For this review, take the finished solid that the model builds, in its own axes (mm). Face numbers are marked on the shaded views. A direction names the side the tool comes from. Give positions to 0.01 mm unless a question says otherwise; leave off trailing zeros. Write each loop counter-clockwise with the first axis right and the second up, starting at its lowest first coordinate (ties: lowest second). Pieces come first, ordered by that corner, then holes.
Q1. We need section D-D (z = -11). Write out the cut boundary in (x, y).
Q2. Machinability: for the marked faces 1, 2 and 3, which of the approach directions +Z, -Z, +X, -X, +Y, -Y give a long, thin tool a straight path to every point of the face, cutting with its end or side? Answer none if there is none.
Q3. We need section B-B (y = 0.95). Write out the cut boundary in (x, z).
Q4. For line 1 (X direction, y = 3.8, z = 0); line 2 (Z direction, x = 31.5, y = 2.6); line 3 (X direction, y = 4.75, z = -11.5), list the stretches that pass through material, from the lowest coordinate up.
Q5. We need section A-A (z = 0). Write out the cut boundary in (x, y).
Q6. Mouldability with a two-part tool opening along Z and no side actions: class the marked faces 4, 5, 6 and 7 as released by +Z, released by -Z, zero draft, split by the parting line, or undercut.
Q7. We need section C-C (x = -24). Write out the cut boundary in (y, z), then the cut area to 3 significant figures.
Q8. Insertion check: P1, Ø2.5, axis at y = 3.5, z = 13, coming from the +X side; P2, Ø1.6, axis at x = 33, y = 2, coming from the +Z side; P3, Ø2, axis at x = 32, y = 3.5, coming from the -Z side. Each pin has a flat end and moves straight along its axis. Give the tip position at first contact, or say it passes through.
```python
from build123d import *

# Parameters (mm, degrees)
SKETCH1_W           = 53
SKETCH1_H           = 40
BOSS_EXTRUDE1_DEPTH = 5
SKETCH2_R           = 1.75
CUT_EXTRUDE1_DEPTH  = 5
SKETCH3_W           = 40
SKETCH3_H           = 5
BOSS_EXTRUDE2_DEPTH = 1
FILLET2_R           = 10
BOSS_EXTRUDE3_DEPTH = 5
SKETCH5_R           = 3
CUT_EXTRUDE2_DEPTH  = 7
FILLET3_R           = 5


with BuildPart() as part:
    # Sketch1 → Boss-Extrude1 (new body)
    with BuildSketch(Plane(origin=(0, 0, 0), x_dir=(1, 0, 0), z_dir=(0, 1, 0))):
        Rectangle(SKETCH1_W, SKETCH1_H)
    extrude(amount=BOSS_EXTRUDE1_DEPTH)

    # Sketch2 → Cut-Extrude1 (cut)
    with BuildSketch(Plane(origin=(0, 5, 0), x_dir=(1, 0, 0), z_dir=(0, 1, 0))):
        with Locations(Location((-24, 10.252098, 0), (0, 0, 270))):
            Circle(SKETCH2_R)
        with Locations(Location((-24, -10.252098, 0), (0, 0, 270))):
            Circle(SKETCH2_R)
    extrude(amount=-CUT_EXTRUDE1_DEPTH, mode=Mode.SUBTRACT)

    # Sketch3 → Boss-Extrude2 (add)
    with BuildSketch(Plane.ZY.offset(26.5)):
        with Locations((0, 2.5)):
            Rectangle(SKETCH3_W, SKETCH3_H)
    extrude(amount=BOSS_EXTRUDE2_DEPTH)

    # Fillet2
    fillet2_edges = [part.edges().sort_by_distance(p)[0] for p in [
        (-27.5, 2.5, -20),
        (-27.5, 2.5, 20),
    ]]
    fillet(fillet2_edges, radius=FILLET2_R)

    # Sketch4 → Boss-Extrude3 (add)
    with BuildSketch(Plane(origin=(0, 5, 0), x_dir=(1, 0, 0), z_dir=(0, 1, 0))):
        with BuildLine():
            Line((26.5, 5), (33.5, 5))
            ThreePointArc((33.5, 5), (38.5, 0), (33.5, -5))
            Line((33.5, -5), (26.5, -5))
            Line((26.5, -5), (26.5, 5))
        make_face()
    extrude(amount=-BOSS_EXTRUDE3_DEPTH)

    # Sketch5 → Cut-Extrude2 (cut)
    with BuildSketch(Plane(origin=(0, 5, 0), x_dir=(1, 0, 0), z_dir=(0, 1, 0))):
        with Locations(Location((33.5, 0, 0), (0, 0, 270))):
            Circle(SKETCH5_R)
    extrude(amount=-CUT_EXTRUDE2_DEPTH, mode=Mode.SUBTRACT)

    # Fillet3
    fillet3_edges = [part.edges().sort_by_distance(p)[0] for p in [
        (26.5, 2.5, 5),
        (26.5, 2.5, -5),
    ]]
    fillet(fillet3_edges, radius=FILLET3_R)


solid = part.part
```
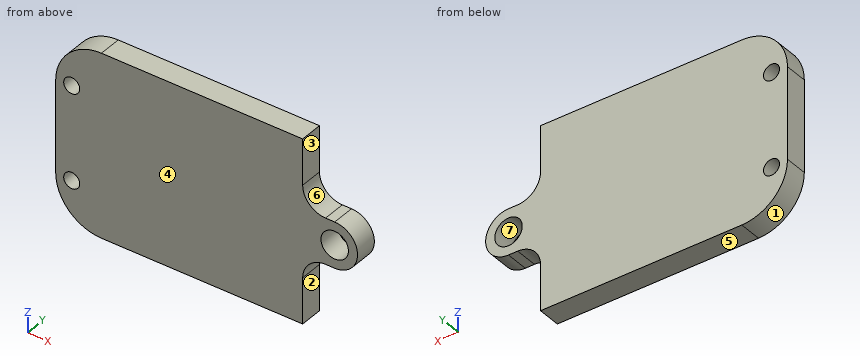
Computed:
1. outline: (-27.45, 0) - (-25.58, 0) - (-25.58, 5) - (-27.45, 5) - close; (-22.42, 0) - (26.5, 0) - (26.5, 5) - (-22.42, 5) - close
2. face 1: -Z, -X, +Y, -Y
2. face 2: -Z, +X, +Y, -Y
2. face 3: +Z, +X, +Y, -Y
3. outline: (-27.5, -10) arc R10 ccw to (-17.5, -20) - (26.5, -20) - (26.5, -10) arc R5 cw to (31.5, -5) - (33.5, -5) arc R5 ccw to (33.5, 5) - (31.5, 5) arc R5 cw to (26.5, 10) - (26.5, 20) - (-17.5, 20) arc R10 ccw to (-27.5, 10) - close; hole circle Ø3.5 at (-24, -10.25); hole circle Ø3.5 at (-24, 10.25); hole circle Ø6 at (33.5, 0)
4. line 1: x = -27.5 to 30.5, 36.5 to 38.5
4. line 2: z = -5 to -2.24, 2.24 to 5
4. line 3: x = -27.39 to -25.23, -22.77 to 26.5
5. outline: (-27.5, 0) - (30.5, 0) - (30.5, 5) - (-27.5, 5) - close; (36.5, 0) - (38.5, 0) - (38.5, 5) - (36.5, 5) - close
6. face 4: zero draft
6. face 5: released by -Z
6. face 6: released by +Z
6. face 7: undercut
7. outline: (0, -17.6) - (5, -17.6) - (5, -12) - (0, -12) - close; (0, -8.5) - (5, -8.5) - (5, 8.5) - (0, 8.5) - close; (0, 12) - (5, 12) - (5, 17.6) - (0, 17.6) - close
7. area: 141 mm2
8. P1: stops at x = 26.5
8. P2: stops at z = 5
8. P3: stops at z = -5.03
